```python
from build123d import *

# Parameters (mm, degrees)
BOSS_EXTRUDE1_DEPTH = 3.175


with BuildPart() as part:
    # Sketch1 → Boss-Extrude1 (new body)
    with BuildSketch(Plane(origin=(38.1, 0, 0), x_dir=(0, 0, -1), z_dir=(1, 0, 0))):
        with BuildLine():
            Line((53.975, 13.934655528), (50.8, 13.934655528))
            Line((50.8, 13.934655528), (50.8, 39.248123167))
            add(Edge.make_bspline(
                [(50.8, 39.248123167), (50.114337, 38.95697122), (45.517089309, 36.98001911), (37.125857024, 33.052669943), (27.830125776, 27.881863583), (20.719091236, 23.242106564), (15.614494654, 19.455138907), (10.786662405, 15.322065366), (6.429542578, 10.752123034), (3.32977957, 6.520652954), (1.7663924, 3.289417246), (1.234577983, 1.629552847), (1.070915718, 0.808496426), (1.022678144, 0.373573946), (1.007771389, 0.114040702), (1.000919428, -0.010571554)],
                knots=[0.920379078, 0.920379078, 0.920379078, 0.920379078, 0.923068011, 0.938443771, 0.95381953, 0.96150741, 0.96919529, 0.97688317, 0.984571049, 0.992258929, 0.996102869, 0.998024839, 0.998985824, 0.999466316, 0.999946809, 0.999946809, 0.999946809, 0.999946809], degree=3))
            add(Edge.make_bspline(
                [(1.000919428, -0.010571554), (1.009921864, -0.277884035), (1.028925425, -0.823363517), (1.10276659, -1.825860568), (1.41675837, -3.59720545), (2.452149912, -7.203198014), (4.557689087, -12.131447527), (7.694251284, -17.873839822), (12.081450574, -25.466402985), (17.732187967, -34.796472344), (24.919918009, -45.768226926), (31.457639598, -54.481002451), (37.047634728, -61.182548528), (42.818130244, -67.680088504), (47.457882264, -72.162847135), (50.8, -74.824969829)],
                knots=[5.1726e-05, 5.1726e-05, 5.1726e-05, 5.1726e-05, 0.001013083, 0.00197444, 0.003897153, 0.00774258, 0.015433433, 0.023124286, 0.030815139, 0.046196845, 0.061578551, 0.076960258, 0.084651111, 0.092341964, 0.107535675, 0.107535675, 0.107535675, 0.107535675], degree=3))
            Line((50.8, -74.824969829), (50.8, -50.696741856))
            Line((50.8, -50.696741856), (53.975, -50.696741856))
            Line((53.975, -50.696741856), (53.975, -25.296741856))
            Line((53.975, -25.296741856), (50.8, -25.296741856))
            Line((50.8, -25.296741856), (50.8, -11.465344472))
            Line((50.8, -11.465344472), (53.975, -11.465344472))
            Line((53.975, -11.465344472), (53.975, 13.934655528))
        make_face()
    extrude(amount=-BOSS_EXTRUDE1_DEPTH)


solid = part.part
```
Input: part model. Units: mm. Frame: model coordinates. A direction names the side the tool comes from. Coordinates: 2 decimals unless noted, no trailing zeros. Answer in a Markdown table with one row per item.
(1) Pin query (flat end, axial travel): P1, Ø1.5, axis at x = 37, z = -37.5, coming from the +Y side; P2, Ø1.5, axis at x = 36, z = -29.5, coming from the +Y side; P3, Ø1.6, axis at x = 36, z = -52, coming from the -Y side. Return the tip coordinate at first contact, or that it passes through.
Model answer:
| item | result |
|---|---|
| P1 | stops at y = 33.46 |
| P2 | stops at y = 29.16 |
| P3 | stops at y = -50.7 |
(2) Material intervals for L1, parallel to Y at x = 35.2, z = -18; L2, parallel to Z at x = 35.2, y = -56; L3, parallel to Y at x = 38.05, z = -26.5, sorted ascending. Write a range as from..to.
Model answer:
| item | result |
|---|---|
| L1 | y = -35.08..21.2 |
| L2 | z = -50.8..-32.78 |
| L3 | y = -47.75..26.94 |
(3) Set-up query: faces 4 (the face through (37, -38, -53.975)), 5 (the face through (37, -18, -50.8)), 6 (the face through (37, -50.697, -52)). Return all of +Z, -Z, +X, -X, +Y, -Y with unobstructed straight access to the full face (end or side cutting, diameter ignored); none if empty.
Model answer:
| item | result |
|---|---|
| face 4 | -Z, +X, -X, +Y, -Y |
| face 5 | -Z, +X, -X |
| face 6 | -Z, +X, -X, -Y |
(4) Mould query, pull axis Y, two halves, no side actions, for faces 1 (the face through (37, -25.297, -52)), 2 (the face through (37, 13.935, -52)), 3 (the face through (37, 26, -50.8)). Classes: pulls with the +Y half, pulls with the -Y half, needs draft (parallel to the pull), parting line crosses it, or undercut.
Model answer:
| item | result |
|---|---|
| face 1 | undercut |
| face 2 | pulls with the +Y half |
| face 3 | needs draft |
